Check sheet for the modelled part. Datum: model origin and axes. Units: mm. Round coordinates to 2 decimals unless told otherwise and drop trailing zeros. Order: outer loops, then holes, each group sorted by start corner. A loop starts at its lowest first (then second) coordinate and runs counter-clockwise, first axis right, second up.
(1) Sectioned sample at A-A, the plane z = 3.8. Enter the section's corners in (x, y).
(2) Sectioned sample at D-D, the plane x = 41.5. Enter the section's corners in (y, z).
(3) Sectioned sample at B-B, the plane z = 0.6. Enter the section's corners in (x, y).
(4) Sectioned sample at C-C, the plane y = 11. Enter the section's corners in (x, z).
(5) Depth check by flat-ended pin: pin 1 (1.7 mm diameter, centred on x = 1.5, y = -2, fed in from +Z); pin 2 (5 mm diameter, centred on x = 33, y = 4.5, fed in from -Z). Enter the tip coordinate at first touch or a pass-through.
(6) Thickness scan on probe 1 along Y at (x, z) = (19.5, 4.05); probe 2 along Y at (x, z) = (36, 2.85). Record the ranges inside material, lowest first.
Autodesk Inventor part; units mm, degrees
ref_plane "YZ Plane" through (0, 0, 0) normal (1, 0, 0) x (0, 1, 0)
ref_plane "XZ Plane" through (0, 0, 0) normal (0, 1, 0) x (-1, 0, 0)
ref_plane "XY Plane" through (0, 0, 0) normal (0, 0, 1) x (1, 0, 0)
sketch "Sketch1" plane through (0, 0, 0) normal (0, 0, 1) x (1, 0, 0)
  circle A0 centre (1.6652, -2.7344) radius 1.1
  circle A1 centre (1.6652, -2.7344) radius 2.5
  circle A2 centre (48.2864, 14.0238) radius 1.1 construction
  point P0 (0, 0)
  dimension "d0" = 5
extrude "Extrusion1" add sketch "Sketch1" along normal blind 2.5
sketch "Sketch2" plane through (1.6652, -2.7344, 2.5) normal (0, 0, 1) x (1, 0, 0)
  circle A0 centre (0, 0) radius 2.5
  circle A1 centre (0, 0) radius 1.1
  circle A2 centre (46.6212, 16.7582) radius 1.1
  circle A3 centre (46.6212, 16.7582) radius 2.5
  circle A4 centre (0, 0) radius 2.5
  line L0 (0.8457, -2.3526) -> (47.4669, 14.4056)
  line L1 (-0.8457, 2.3526) -> (45.7756, 19.1109)
  point P0 (-1.6652, 2.7344)
  point P1 (0.8457, -2.3526)
  dimension "d4" = 5
extrude "Extrusion2" add sketch "Sketch2" along normal blind 2.5
sketch "Sketch3" plane through (0.8195, -0.3818, 5) normal (-0.3382652, 0.9410508, 0) x (0.9410508, 0.3382652, 0)
  line L0 (49.5417, 2.5) -> (0, 2.5)
  line L1 (0, 2.5) -> (0, 0)
  line L2 (49.5417, 0) -> (0, 0)
  line L3 (49.5417, 2.5) -> (49.5417, 0)
  line L4 (0, 2.5) -> (0, 2.5)
  line L5 (0, 2.5) -> (0, 0)
  line L6 (0, 0) -> (0, 0)
  line L7 (0, 2.5) -> (0, 0)
  line L8 (-2.5, 5) -> (2.5, 5)
  line L9 (-2.5, 0) -> (0, 0)
  line L10 (-2.5, 5) -> (-2.5, 0)
  line L11 (-2.5, 5) -> (2.5, 5)
  line L12 (2.5, 5) -> (16.6782, 2.5)
  line L13 (0, 2.5) -> (49.5417, 2.5)
  line L14 (2.5, 5) -> (2.5, 2.5)
  line L15 (0, 0) -> (49.5417, 0)
  line L16 (0, 2.5) -> (2.5, 2.5)
  line L17 (16.6782, 0) -> (2.5, 2.5)
  point P0 (-0.6421, 5)
  point P1 (16.6782, 2.5)
  dimension "d7" = 10
extrude "Extrusion3" add sketch "Sketch3" against normal blind 5 contours L0 L14 L12
sketch "Sketch4" plane through (3.1722, 0.4639, 0) normal (-0.9410508, -0.3382652, 0) x (0, 0, 1)
  line L0 (0, -2.5) -> (2.5, -2.5)
  line L1 (2.5, 0) -> (2.5, -2.5)
  line L2 (0, 0) -> (2.5, 0)
  line L3 (0, 0) -> (0, -2.5)
  line L4 (0, -2.5) -> (0, -5)
  line L5 (2.5, -5) -> (0, -5)
  line L6 (2.5, -2.5) -> (2.5, -5)
  point P0 (0, 0.6365)
extrude "Extrusion4" add sketch "Sketch4" along normal up to surface
sketch "Sketch5" plane through (0.8195, -0.3818, 5) normal (-0.3382652, 0.9410508, 0) x (0.9410508, 0.3382652, 0)
  line L0 (0, 5) -> (0, 0)
  line L1 (0, 0) -> (0, 0)
  line L2 (0, 5) -> (0, 0)
  line L3 (0, 5) -> (0, 5)
  line L4 (49.5417, 2.5) -> (16.6782, 2.5)
  line L5 (16.6782, 2.5) -> (2.5, 5)
  line L6 (2.5, 5) -> (0, 5)
  line L7 (0, 5) -> (0, 0)
  line L8 (49.5417, 0) -> (0, 0)
  line L9 (49.5417, 2.5) -> (49.5417, 0)
  line L10 (-1.1, 0) -> (-1.1, 5)
  line L11 (-2.5, 5) -> (-2.5, 0)
  line L12 (-2.5, 0) -> (0, 0)
  line L13 (-2.5, 5) -> (0, 5)
  line L14 (-2.5, 2.5) -> (2.5, 2.5)
  line L15 (2.5, 2.5) -> (16.6782, 0)
  point P0 (-0.6421, 5)
extrude "Extrusion5" cut sketch "Sketch5" against normal up to next contours L14 L15 L8 L0 | L0 L12 L10 L14 | L10 L12 L11 L14
properties part number "Dedo_3"
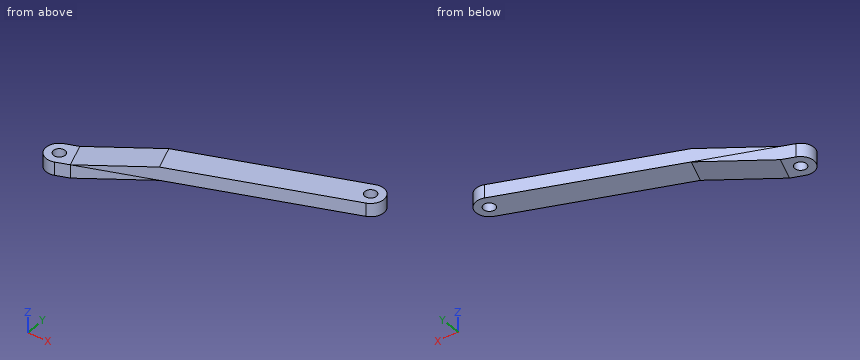
Derived:
1. outline: (10.11, 2.96) - (11.8, -1.75) - (49.13, 11.67) arc R2.5 ccw to (47.44, 16.38) - close; hole circle Ø2.2 at (48.29, 14.02)
2. outline: (8.93, 2.5) - (14.24, 2.5) - (14.24, 5) - (8.93, 5) - close
3. outline: (0.82, -0.38) arc R2.5 ccw to (2.51, -5.09) - (8.07, -3.09) - (6.37, 1.61) - close; hole circle Ø2.2 at (1.67, -2.73)
4. outline: (32.48, 2.5) - (47.26, 2.5) - (47.26, 5) - (32.48, 5) - close
5. pin 1: stops at z = 2.5
5. pin 2: stops at z = 2.5
6. probe 1: y = 1.02 to 6.33
6. probe 2: y = 6.95 to 12.26
